```python
from build123d import *

# Parameters (mm, degrees)
F0_R     = 30
F1_DEPTH = 40
F3_DEPTH = 32
F5_DEPTH = 25


with BuildPart() as f1:
    # F0 (on Front) → F1 (new body, symmetric)
    with BuildSketch(Plane.XZ):
        Circle(F0_R)
    extrude(amount=F1_DEPTH, both=True)

    # F2 (on face) → F3 (cut)
    with BuildSketch(Plane.XZ.offset(40)):
        with BuildLine():
            Line((28.2842712475, 10), (-28.2842712475, 10))
            ThreePointArc((-28.2842712475, 10), (-30, 0), (-28.2842712475, -10))
            Line((-28.2842712475, -10), (28.2842712475, -10))
            ThreePointArc((28.2842712475, -10), (29.5679567896, -5.0730593618), (30, 0))
            ThreePointArc((30, 0), (29.5679567896, 5.0730593618), (28.2842712475, 10))
        make_face()
    extrude(amount=-F3_DEPTH, mode=Mode.SUBTRACT)

    # F4 (on face) → F5 (cut)
    with BuildSketch(Plane(origin=(0, 40, 0), x_dir=(-1, 0, 0), z_dir=(0, 1, 0))):
        with BuildLine():
            Line((10.5825905188, 28.0714940449), (10.5825905188, -28.0714940449))
            ThreePointArc((10.5825905188, -28.0714940449), (24.6726337828, -17.0663746067), (30, 0))
            ThreePointArc((30, 0), (24.6726337828, 17.0663746067), (10.5825905188, 28.0714940449))
        make_face()
        with BuildLine():
            ThreePointArc((-10.5825905188, 28.0714940449), (-30, 0), (-10.5825905188, -28.0714940449))
            Line((-10.5825905188, -28.0714940449), (-10.5825905188, 28.0714940449))
        make_face()
    extrude(amount=-F5_DEPTH, mode=Mode.SUBTRACT)


solid = f1.part
```
For this review, take the finished solid that the model builds, in its own axes (mm). A direction names the side the tool comes from. Give positions to 0.01 mm unless a question says otherwise; leave off trailing zeros. Write each loop counter-clockwise with the first axis right and the second up, starting at its lowest first coordinate (ties: lowest second). Pieces come first, ordered by that corner, then holes.
Item 1: Take a section at A-A (x = 0). Give the boundary of the cut face in (y, z).
Item 2: Take a section at C-C (z = -18). Give the boundary of the cut face in (x, y).
Item 3: Wall thickness on probe 1 along Y at (x, z) = (-12.5, 16.5); probe 2 along Y at (x, z) = (4.5, -8.5); probe 3 along Z at (x, y) = (0, -3): over which ranges is each line inside the solid? List them lowest first.
Item 4: Take a section at B-B (y = -12). Give the boundary of the cut face in (x, z).
Item 5: Take a section at D-D (y = -1.5). Give the boundary of the cut face in (x, z).
Item 6: Machinability: for faces 5 (the face through (0, 40, 0)), 6 (the face through (0, -24, -10)), 7 (the face through (0, -40, 18)), 8 (the face through (-18, 15, 0)), 9 (the face through (10.583, 28, 0)), which of the approach directions +Z, -Z, +X, -X, +Y, -Y give a long, thin tool a straight path to every point of the face, cutting with its end or side? Answer none if there is none.
Item 7: Insertion check: P1, Ø7.5, axis at y = 33, z = 1.5, coming from the -X side; P2, Ø12.5, axis at y = 22, z = 6, coming from the +X side; P3, Ø10, axis at y = 19.5, z = 8, coming from the -X side. Each pin has a flat end and moves straight along its axis. Give the tip position at first contact, or say it passes through.
Item 8: The part is to be moulded in two halves that separate along Z. For faces 1 (the face through (-24, -9, -18)), 2 (the face through (18, 15, 0)), 3 (the face through (0, -24, 10)), 4 (the face through (0, -8, 0)), say which applies: +Z half, -Z half, draft (parallel to the pull), parting line (faces both ways), or undercut.
Established:
1. outline: (-40, -30) - (40, -30) - (40, 30) - (-40, 30) - (-40, 10) - (-8, 10) - (-8, -10) - (-40, -10) - close
2. outline: (-24, -40) - (24, -40) - (24, 15) - (10.58, 15) - (10.58, 40) - (-10.58, 40) - (-10.58, 15) - (-24, 15) - close
3. probe 1: y = -40 to 15
3. probe 2: y = -8 to 40
3. probe 3: z = -30 to 30
4. outline: (-28.28, -10) arc R30 ccw to (28.28, -10) - close; (-28.28, 10) - (28.28, 10) arc R30 ccw to start
5. outline: circle Ø60 at (0, 0)
6. face 5: +Z, -Z, +X, -X, +Y
6. face 6: +X, -X, -Y
6. face 7: +Z, -Z, +X, -X, -Y
6. face 8: +Z, -Z, -X, +Y
6. face 9: +Z, -Z, +X, +Y
7. P1: stops at x = -10.58
7. P2: stops at x = 10.58
7. P3: stops at x = -29.43
8. face 1: parting line
8. face 2: draft
8. face 3: undercut
8. face 4: undercut
